Input: part model. Units: mm. Frame: model coordinates. A direction names the side the tool comes from. Give positions to 0.01 mm unless a question says otherwise; leave off trailing zeros. Loops run counter-clockwise (first coordinate to the right, second up) from the corner with the lowest first, then second, coordinate; pieces in that order, holes last. Notation, with made-up numbers: M -13,47.5 L 11,47.5 A26 cw 11,72.5 Z; hole C -35,-35 d11. An arc over 180 degrees is marked long. Answer as a JSON object with one key per item and string values. Group by question number.
```python
from build123d import *

# Parameters (mm, degrees)
BOSS_EXTRUDE1_DEPTH = 16
CUT_EXTRUDE1_DEPTH  = 16
SKETCH5_R           = 10
BOSS_EXTRUDE2_DEPTH = 12
FILLET1_R           = 2


with BuildPart() as part:
    # Sketch2 → Boss-Extrude1 (new body)
    with BuildSketch(Plane(origin=(0, 0, 0), x_dir=(1, 0, 0), z_dir=(0, 1, 0))):
        with BuildLine():
            Line((37, 22), (-59, 22))
            Line((-59, 22), (-59, -22))
            Line((-59, -22), (37, -22))
            ThreePointArc((37, -22), (59, 0), (37, 22))
        make_face()
    extrude(amount=BOSS_EXTRUDE1_DEPTH)

    # Sketch3 → Cut-Extrude1 (cut)
    with BuildSketch(Plane(origin=(0, 16, 0), x_dir=(1, 0, 0), z_dir=(0, 1, 0))):
        with BuildLine():
            Line((37, -8), (13, -8))
            ThreePointArc((13, -8), (5, 0), (13, 8))
            Line((13, 8), (37, 8))
            ThreePointArc((37, 8), (45, 0), (37, -8))
        make_face()
    extrude(amount=-CUT_EXTRUDE1_DEPTH, mode=Mode.SUBTRACT)

    # Sketch5 → Boss-Extrude2 (add)
    with BuildSketch(Plane.XY.offset(22)):
        with BuildLine():
            Line((-59, 16), (-11, 16))
            Line((-11, 16), (-11, 36.094530012))
            ThreePointArc((-11, 36.094530012), (-35, 64.315688266), (-59, 36.094530012))
            Line((-59, 36.094530012), (-59, 16))
        make_face()
        with Locations((-35, 40)):
            Circle(SKETCH5_R, mode=Mode.SUBTRACT)
    boss_extrude2 = extrude(amount=-BOSS_EXTRUDE2_DEPTH)

    # Mirror1: Boss-Extrude2 across plane
    add(boss_extrude2.mirror(Plane.XY))

    # Fillet1
    fillet1_edges = [part.edges().sort_by_distance(p)[0] for p in [
        (-11, 16, 16),
        (-35, 16, 10),
        (-35, 16, -10),
        (-11, 16, -16),
    ]]
    fillet(fillet1_edges, radius=FILLET1_R)


solid = part.part
```
1. Reachability of faces 4 (the flat face through (-30, 31, -10)), 5 (the flat face through (-11, 27, 16)), 6 (the cylindrical face through (45, 8, 0)) from +Z, -Z, +X, -X, +Y, -Y: full face, straight path, thin tool, end or side. Return the list, or none.
2. Section C-C (z = -1). Output: boundary loops of the cut face in (x, y).
3. Section A-A (x = 24). Output: boundary loops of the cut face in (y, z), then the cut area to 3 significant figures.
4. Section D-D (y = 40). Output: boundary loops of the cut face in (x, z), then the cut area to 3 significant figures.
5. Section B-B (y = 11). Output: boundary loops of the cut face in (x, z), then the cut area to 3 significant figures.
6. First-contact query: P1, Ø1.5, axis at x = 44, z = 1, coming from the -Y side; P2, Ø6, axis at y = 24, z = -16.5, coming from the +X side; P3, Ø8, axis at x = 5.5, z = -15, coming from the +Y side; P4, Ø22, axis at x = -10, z = 2.5, coming from the +Y side. Flat tips, straight axial feed; report the tip coordinate or a pass-through.
7. Material intervals for L1, parallel to Y at x = -35, z = 13.25; L2, parallel to Z at x = 27.5, y = 15.5; L3, parallel to Z at x = -23, y = 44, sorted ascending.
8. Mould query, pull axis Y, two halves, no side actions, for faces 1 (the flat face through (-23, 25, -22)), 2 (the flat face through (-1, 16, 0)), 3 (the cylindrical face through (-37.17, 30.24, -16.08)). Classes: pulls with the +Y half, pulls with the -Y half, needs draft (parallel to the pull), parting line crosses it, or undercut.
Geometry results:
{
 "1": {"face 4": "+X, -X, +Y", "face 5": "+Z, -Z, +X", "face 6": "+Y, -Y"},
 "2": {"outline": "M -59,0 L 5.06,0 L 5.06,16 L -59,16 Z; M 44.94,0 L 58.98,0 L 58.98,16 L 44.94,16 Z"},
 "3": {"outline": "M 0,-22 L 16,-22 L 16,-8 L 0,-8 Z; M 0,8 L 16,8 L 16,22 L 0,22 Z", "area": "448 mm2"},
 "4": {"outline": "M -59.32,-22 L -45,-22 L -45,-10 L -59.32,-10 Z; M -59.32,10 L -45,10 L -45,22 L -59.32,22 Z; M -25,-22 L -10.68,-22 L -10.68,-10 L -25,-10 Z; M -25,10 L -10.68,10 L -10.68,22 L -25,22 Z", "area": "687 mm2"},
 "5": {"outline": "M -59,-22 L 37,-22 A22 ccw 37,22 L -59,22 Z; hole M 13,-8 L 37,-8 A8 ccw 37,8 L 13,8 A8 ccw Z", "area": "4,400 mm2"},
 "6": {"P1": "through", "P2": "x = -11", "P3": "y = 16", "P4": "y = 57.43"},
 "7": {"L1": "0 to 30, 50 to 64.32", "L2": "-22 to -8, 8 to 22", "L3": "-22 to -10, 10 to 22"},
 "8": {"face 1": "needs draft", "face 2": "pulls with the +Y half", "face 3": "undercut"}
}
